```python
from build123d import *

# Parameters (mm, degrees)
SKETCH1_R           = 132.01
BOSS_EXTRUDE1_DEPTH = 3
CUT_EXTRUDE1_START  = -3
CUT_EXTRUDE1_DEPTH  = 4
CIRPATTERN1_COUNT   = 8
SKETCH7_W           = 3
SKETCH7_H           = 5
CUT_EXTRUDE4_DEPTH  = 3
CIRPATTERN2_COUNT   = 8
SKETCH8_R           = 102.01
CUT_EXTRUDE6_DEPTH  = 10


with BuildPart() as part:
    # Sketch1 → Boss-Extrude1 (new body)
    with BuildSketch(Plane(origin=(0, 0, 0), x_dir=(1, 0, 0), z_dir=(0, 1, 0))):
        Circle(SKETCH1_R)
    extrude(amount=BOSS_EXTRUDE1_DEPTH)

    # Sketch2 → Cut-Extrude1 (cut)
    with BuildSketch(Plane(origin=(0, 3, 0), x_dir=(1, 0, 0), z_dir=(0, 1, 0)).offset(CUT_EXTRUDE1_START)):
        Polygon((-1.5, 733.700659415), (-1.5, 132.001477643), (-1.5, 122.001477643), (1.5, 122.001477643), (1.5, 132.001477643), (1.5, 733.700659415), (1.5, 1937.099022959), (-1.5, 1937.099022959), align=None)
    cut_extrude1 = extrude(amount=CUT_EXTRUDE1_DEPTH, mode=Mode.SUBTRACT)

    # CirPattern1: Cut-Extrude1 ×8 about axis
    cirpattern1_axis = Axis((0, 0, 0), (0, -1, 0))
    for i in range(1, CIRPATTERN1_COUNT):
        add(cut_extrude1.rotate(cirpattern1_axis, i * 360 / CIRPATTERN1_COUNT), mode=Mode.SUBTRACT)

    # Sketch7 → Cut-Extrude4 (cut)
    with BuildSketch(Plane(origin=(0, 3, 0), x_dir=(1, 0, 0), z_dir=(0, 1, 0))):
        with Locations((-3.5, 118.501477643)):
            Rectangle(SKETCH7_W, SKETCH7_H)
        with Locations((3.5, 118.501477643)):
            Rectangle(SKETCH7_W, SKETCH7_H)
    cut_extrude4 = extrude(amount=-CUT_EXTRUDE4_DEPTH, mode=Mode.SUBTRACT)

    # CirPattern2: Cut-Extrude4 ×8 about axis
    cirpattern2_axis = Axis((0, 0, 0), (0, 1, 0))
    for i in range(1, CIRPATTERN2_COUNT):
        add(cut_extrude4.rotate(cirpattern2_axis, i * 360 / CIRPATTERN2_COUNT), mode=Mode.SUBTRACT)

    # Sketch8 → Cut-Extrude6 (cut)
    with BuildSketch(Plane(origin=(0, 3, 0), x_dir=(1, 0, 0), z_dir=(0, 1, 0))):
        Circle(SKETCH8_R)
    extrude(amount=-CUT_EXTRUDE6_DEPTH, mode=Mode.SUBTRACT)


solid = part.part
```
Work out the finished part from the listing and answer in its coordinate system (mm). A direction names the side the tool comes from. Round coordinates to 2 decimals unless told otherwise and drop trailing zeros. Loops run counter-clockwise (first coordinate to the right, second up) from the corner with the lowest first, then second, coordinate; pieces in that order, holes last. Notation, with made-up numbers: M 79,39 L 86,39 A21 ccw 86,70 Z; hole C 89.25,70 d10. An arc over 180 degrees is marked long. One line per question, with ' | ' between items.
Q1. Consider line 1 along Z through (x, y) = (0, 1.8); line 2 along X through (y, z) = (1.3, -43). Determine where each line is inside the solid, lowest interval first. Write a range as from..to.
Conclusion:
line 1: z = -122..-102.01, 102.01..122 | line 2: x = -124.81..-92.5, 92.5..124.81
Q2. The mould has two halves that part along Z. Classify faces 1 (the flat face through (-90.81, 1.48, 88.69)), 2 (the flat face through (38, 0, 97)), 3 (the cylindrical face through (49.866, 1.479, 122.229)): +Z half, -Z half, draft (parallel to the pull), parting line (faces both ways), or undercut.
Conclusion:
face 1: undercut | face 2: draft | face 3: +Z half
Q3. Each of these flat-tipped pins is pushed along its axis until it touches: pin 1 Ø1.5 at (y, z) = (1.5, 0) entering from +X; pin 2 Ø1.5 at (x, y) = (-119, 1) entering from -Z; pin 3 Ø0.9 at (x, y) = (-3.5, 1) entering from +Z; pin 4 Ø2 at (x, z) = (-104, -20) entering from -Y. Where does it stop, or does it pass through?
Conclusion:
pin 1: stops at x = 122 | pin 2: stops at z = -58.68 | pin 3: stops at z = 131.97 | pin 4: stops at y = 0
Q4. Find section C-C, the plane y = 2.25. State how many separate pieces and enclosed holes the cut face has, then the cut area to 3 significant figures.
Conclusion:
separate pieces: 1 | enclosed holes: 17 | area: 21,600 mm2
Q5. Find section D-D, the plane z = 111.5. Give the vertices of the cut face in (x, y).
Conclusion:
outline: M -70.67,0 L 70.67,0 L 70.67,3 L -70.67,3 Z
Q6. A tool of negligible diameter and unlimited length cuts with its end or side. For faces 4 (the cylindrical face through (-121.69, 1.48, -51.17)), 5 (the flat face through (90.81, 1.48, -88.69)), from which of +Z, -Z, +X, -X, +Y, -Y can it reach the whole face along a straight path? Write none if from no direction.
Conclusion:
face 4: -Z, -X, +Y, -Y | face 5: +Y, -Y
Q7. Find section A-A, the plane z = 37. Give the vertices of the cut face in (x, y).
Conclusion:
outline: M -126.72,0 L -95.06,0 L -95.06,3 L -126.72,3 Z; M 95.06,0 L 126.72,0 L 126.72,3 L 95.06,3 Z
Q8. Find section B-B, the plane x = 37. Give the vertices of the cut face in (y, z), then the cut area to 3 significant figures.
Conclusion:
outline: M 0,-126.72 L 3,-126.72 L 3,-95.06 L 0,-95.06 Z; M 0,95.06 L 3,95.06 L 3,126.72 L 0,126.72 Z | area: 190 mm2
